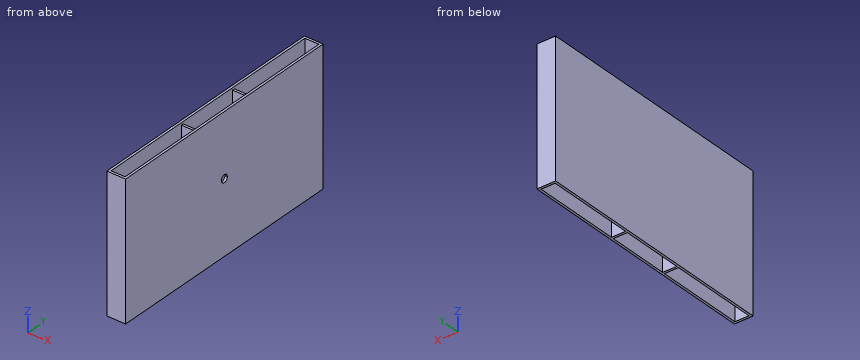
from build123d import *

# Parameters (mm, degrees)
F0_W     = 152.4
F0_H     = 2032
F0_W_2   = 114.3
F0_H_2   = 1993.9
F1_DEPTH = 1098.55
F3_DEPTH = 25.4
F4_W     = 19.05
F4_H     = 1079.5
F5_DEPTH = 114.3


with BuildPart() as f1:
    # F0 (on Top) → F1 (new body)
    with BuildSketch(Plane.XY):
        Rectangle(F0_W, F0_H)
        Rectangle(F0_W_2, F0_H_2, mode=Mode.SUBTRACT)
    extrude(amount=F1_DEPTH)

    # F2 (on face) → F3 (cut)
    with BuildSketch(Plane.YZ.offset(76.2)):
        with BuildLine():
            ThreePointArc((30.226, 590.55), (21.37301, 611.92301), (0, 620.776))
            ThreePointArc((0, 620.776), (-21.37301, 569.17699), (30.226, 590.55))
        make_face()
    extrude(amount=-F3_DEPTH, mode=Mode.SUBTRACT)

    # F4 (on face) → F5 (join)
    with BuildSketch(Plane.YZ.offset(-57.15)):
        with Locations((-263.525, 539.75)):
            Rectangle(F4_W, F4_H)
        with Locations((263.525, 539.75)):
            Rectangle(F4_W, F4_H)
    extrude(amount=F5_DEPTH)


solid = f1.part
Work out the finished part from the listing and answer in its coordinate system (mm). Give positions to 0.01 mm unless a question says otherwise; leave off trailing zeros. Write each loop counter-clockwise with the first axis right and the second up, starting at its lowest first coordinate (ties: lowest second). Pieces come first, ordered by that corner, then holes. Notation, with made-up numbers: (12.25, -34) - (60.25, -34) arc R12 cw to (60.25, -18) - close; hole circle Ø1 at (-36, 20). An arc over 180 degrees is marked (long way). One line per item, written item: value. Start each with the question number.
1. Given pin 1 (5.5 mm diameter, centred on x = 7.5, y = 263.5, fed in from +Z); pin 2 (2 mm diameter, centred on x = -54.5, y = -642, fed in from +Z), each flat-ended and moving along its own axis, determine where each tip first touches the part or whether it passes through.
2. Consider probe 1 along Y at (x, z) = (-22.5, 370); probe 2 along X at (y, z) = (429.5, 1032); probe 3 along Z at (x, y) = (68, 0). Determine where each line is inside the solid, lowest interval first.
3. Find section A-A (x = -34). Write down the section's boundary in (y, z), then the cut area to 3 significant figures.
4. Find section C-C (y = -119). Write down the section's boundary in (x, z), then the cut area to 3 significant figures.
5. Find section B-B (z = 771). Write down the section's boundary in (x, y).
Geometry results:
1. pin 1: z = 1079.5
1. pin 2: through
2. probe 1: -1016 to -996.95, -273.05 to -254, 254 to 273.05, 996.95 to 1016
2. probe 2: -76.2 to -57.15, 57.15 to 76.2
2. probe 3: 0 to 560.32, 620.78 to 1098.55
3. outline: (-1016, 0) - (-996.95, 0) - (-996.95, 1098.55) - (-1016, 1098.55) - close; (-273.05, 0) - (-254, 0) - (-254, 1079.5) - (-273.05, 1079.5) - close; (254, 0) - (273.05, 0) - (273.05, 1079.5) - (254, 1079.5) - close; (996.95, 0) - (1016, 0) - (1016, 1098.55) - (996.95, 1098.55) - close
3. area: 83,000 mm2
4. outline: (-76.2, 0) - (-57.15, 0) - (-57.15, 1098.55) - (-76.2, 1098.55) - close; (57.15, 0) - (76.2, 0) - (76.2, 1098.55) - (57.15, 1098.55) - close
4. area: 41,900 mm2
5. outline: (-76.2, -1016) - (76.2, -1016) - (76.2, 1016) - (-76.2, 1016) - close; hole (-57.15, -996.95) - (57.15, -996.95) - (57.15, -273.05) - (-57.15, -273.05) - close; hole (-57.15, -254) - (57.15, -254) - (57.15, 254) - (-57.15, 254) - close; hole (-57.15, 273.05) - (57.15, 273.05) - (57.15, 996.95) - (-57.15, 996.95) - close
